Geometry: see drawing. Coordinates: mm, zero at the bounding-box minimum. Give positions to 0.01 mm unless a question says otherwise; leave off trailing zeros. Write each loop counter-clockwise with the first axis right and the second up, starting at its lowest first coordinate (ties: lowest second). Pieces come first, ordered by that corner, then holes.
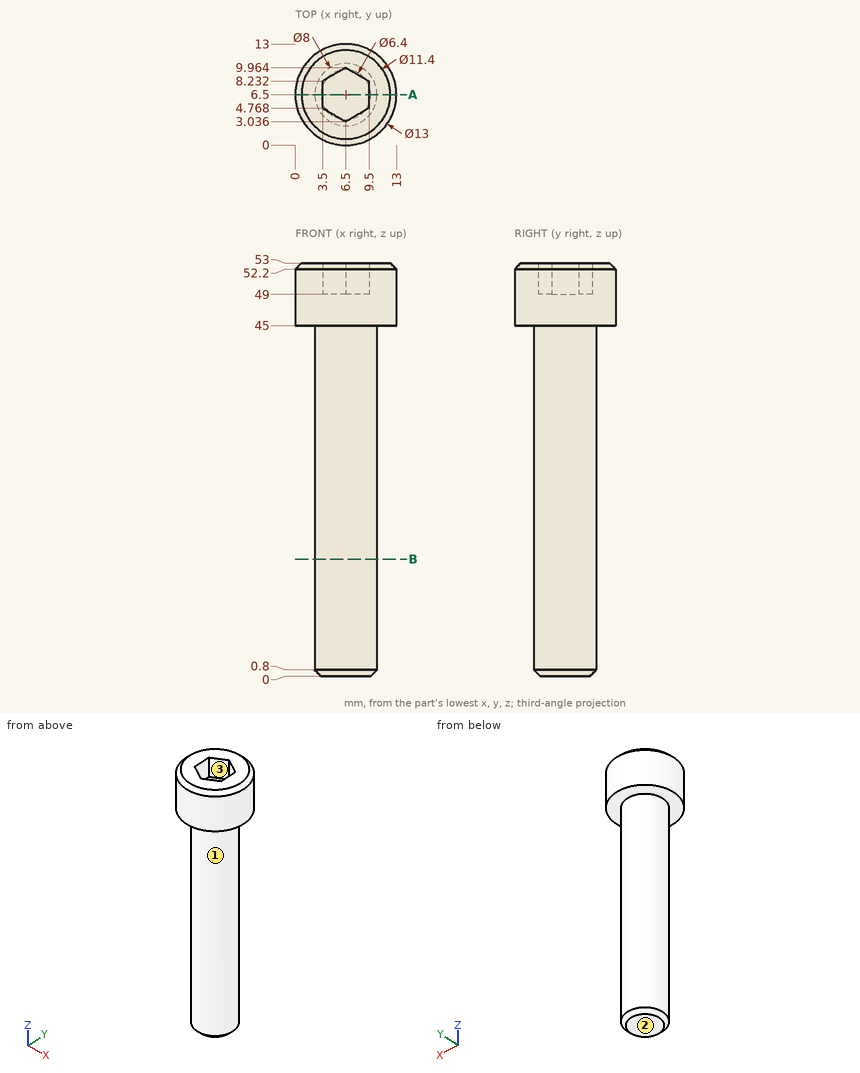
1. Line query: probe 1 along Z at (x, y) = (10, 8.5); probe 2 along Z at (x, y) = (8, 5.75); probe 3 along Y at (x, z) = (6.75, 30.5). Output: solid intervals per line, ascending.
2. Pull-direction query (X, two-part tool) for the marked faces 1, 2 and 3; classes: pulls with the +X half, pulls with the -X half, needs draft (parallel to the pull), parting line crosses it, or undercut.
3. Section query B-B (z = 15). Return loops of the section in (x, y), plus the area to 3 significant figures.
4. Pin query (flat end, axial travel): P1, Ø3, axis at x = 6.5, y = 5.5, coming from the +Z side; P2, Ø6, axis at y = 9, z = 17.5, coming from the +X side; P3, Ø1.5, axis at y = 8.5, z = 27, coming from the +X side. Return the tip coordinate at first contact, or that it passes through.
5. Section query A-A (y = 6.5). Return loops of the section in (x, z), plus the area to 3 significant figures.
The answers:
1. probe 1: z = 45 to 53
1. probe 2: z = 0 to 49
1. probe 3: y = 2.51 to 10.49
2. face 1: parting line crosses it
2. face 2: needs draft
2. face 3: undercut
3. outline: circle Ø8 at (6.5, 6.5)
3. area: 50.3 mm2
4. P1: stops at z = 49
4. P2: stops at x = 10.5
4. P3: stops at x = 10.3
5. outline: (0, 45) - (2.5, 45) - (2.5, 0.8) - (3.3, 0) - (9.7, 0) - (10.5, 0.8) - (10.5, 45) - (13, 45) - (13, 52.2) - (12.2, 53) - (9.5, 53) - (9.5, 49) - (3.5, 49) - (3.5, 53) - (0.8, 53) - (0, 52.2) - close
5. area: 439 mm2
